Geometry check sheet. Reference: the model listing, model coordinates, mm. A direction names the side the tool comes from. Give positions to 0.01 mm unless a question says otherwise; leave off trailing zeros. Write each loop counter-clockwise with the first axis right and the second up, starting at its lowest first coordinate (ties: lowest second). Pieces come first, ordered by that corner, then holes. Notation, with made-up numbers: M 7.5,50 L 56.5,50 A23 ccw 56.5,78 Z; hole C 46,41.5 d10. An arc over 180 degrees is marked long. Write each question's results on one line, items separated by ' | '.
Autodesk Inventor part; units mm, degrees
ref_plane "YZ Plane" through (0, 0, 0) normal (1, 0, 0) x (0, 1, 0)
ref_plane "XZ Plane" through (0, 0, 0) normal (0, 1, 0) x (-1, 0, 0)
ref_plane "XY Plane" through (0, 0, 0) normal (0, 0, 1) x (1, 0, 0)
sketch "Sketch4" plane through (0, 0, 0) normal (0, 0, 1) x (1, 0, 0)
  line L0 (0, 500) -> (50, 500)
  line L1 (50, 500) -> (50, 0)
  line L2 (50, 0) -> (0, 0)
  line L3 (0, 0) -> (0, 500)
  dimension "d31" = 50
  dimension "d32" = 500
extrude "Extrusion1" add sketch "Sketch4" along normal blind 18.55
sketch "Sketch5" plane through (0, 0, 18.55) normal (0, 0, 1) x (1, 0, 0)
  line L0 (50, 500) -> (0, 500)
  line L1 (10, 500) -> (40, 500)
  line L2 (40, 500) -> (40, 537.1)
  line L3 (40, 537.1) -> (10, 537.1)
  line L4 (10, 537.1) -> (10, 500)
  line L5 (0, 500) -> (0, 0)
  line L6 (50, 0) -> (50, 500)
  dimension "d46" = 10
  dimension "d47" = 10
  dimension "d48" = 37.1
extrude "Extrusion2" add sketch "Sketch5" against normal blind 18.55
sketch "Sketch6" plane through (0, 0, 18.55) normal (0, 0, 1) x (1, 0, 0)
  line L0 (50, 500) -> (65, 491.3397)
  line L1 (65, 491.3397) -> (65, 486.3397)
  line L2 (65, 486.3397) -> (50, 486.3397)
  line L3 (50, 500) -> (40, 500)
  line L4 (40, 500) -> (50, 500)
  line L5 (50, 500) -> (50, 486.3397)
  line L6 (50, 0) -> (50, 500)
  line L7 (50, 475) -> (65, 466.3397)
  line L8 (65, 466.3397) -> (65, 461.3397)
  line L9 (65, 461.3397) -> (50, 461.3397)
  line L10 (50, 475) -> (50, 461.3397)
  line L11 (50, 450) -> (65, 441.3397)
  line L12 (65, 441.3397) -> (65, 436.3397)
  line L13 (65, 436.3397) -> (50, 436.3397)
  line L14 (50, 450) -> (50, 436.3397)
  line L15 (50, 425) -> (65, 416.3397)
  line L16 (65, 416.3397) -> (65, 411.3397)
  line L17 (65, 411.3397) -> (50, 411.3397)
  line L18 (50, 425) -> (50, 411.3397)
  line L19 (50, 400) -> (65, 391.3397)
  line L20 (65, 391.3397) -> (65, 386.3397)
  line L21 (65, 386.3397) -> (50, 386.3397)
  line L22 (50, 400) -> (50, 386.3397)
  line L23 (50, 375) -> (65, 366.3397)
  line L24 (65, 366.3397) -> (65, 361.3397)
  line L25 (65, 361.3397) -> (50, 361.3397)
  line L26 (50, 375) -> (50, 361.3397)
  line L27 (50, 350) -> (65, 341.3397)
  line L28 (65, 341.3397) -> (65, 336.3397)
  line L29 (65, 336.3397) -> (50, 336.3397)
  line L30 (50, 350) -> (50, 336.3397)
  line L31 (50, 325) -> (65, 316.3397)
  line L32 (65, 316.3397) -> (65, 311.3397)
  line L33 (65, 311.3397) -> (50, 311.3397)
  line L34 (50, 325) -> (50, 311.3397)
  line L35 (50, 300) -> (65, 291.3397)
  line L36 (65, 291.3397) -> (65, 286.3397)
  line L37 (65, 286.3397) -> (50, 286.3397)
  line L38 (50, 300) -> (50, 286.3397)
  line L39 (50, 275) -> (65, 266.3397)
  line L40 (65, 266.3397) -> (65, 261.3397)
  line L41 (65, 261.3397) -> (50, 261.3397)
  line L42 (50, 275) -> (50, 261.3397)
  line L43 (50, 250) -> (65, 241.3397)
  line L44 (65, 241.3397) -> (65, 236.3397)
  line L45 (65, 236.3397) -> (50, 236.3397)
  line L46 (50, 250) -> (50, 236.3397)
  line L47 (50, 225) -> (65, 216.3397)
  line L48 (65, 216.3397) -> (65, 211.3397)
  line L49 (65, 211.3397) -> (50, 211.3397)
  line L50 (50, 225) -> (50, 211.3397)
  line L51 (50, 200) -> (65, 191.3397)
  line L52 (65, 191.3397) -> (65, 186.3397)
  line L53 (65, 186.3397) -> (50, 186.3397)
  line L54 (50, 200) -> (50, 186.3397)
  line L55 (50, 175) -> (65, 166.3397)
  line L56 (65, 166.3397) -> (65, 161.3397)
  line L57 (65, 161.3397) -> (50, 161.3397)
  line L58 (50, 175) -> (50, 161.3397)
  line L59 (50, 150) -> (65, 141.3397)
  line L60 (65, 141.3397) -> (65, 136.3397)
  line L61 (65, 136.3397) -> (50, 136.3397)
  line L62 (50, 150) -> (50, 136.3397)
  line L63 (50, 125) -> (65, 116.3397)
  line L64 (65, 116.3397) -> (65, 111.3397)
  line L65 (65, 111.3397) -> (50, 111.3397)
  line L66 (50, 125) -> (50, 111.3397)
  line L67 (50, 100) -> (65, 91.3397)
  line L68 (65, 91.3397) -> (65, 86.3397)
  line L69 (65, 86.3397) -> (50, 86.3397)
  line L70 (50, 100) -> (50, 86.3397)
  line L71 (50, 75) -> (65, 66.3397)
  line L72 (65, 66.3397) -> (65, 61.3397)
  line L73 (65, 61.3397) -> (50, 61.3397)
  line L74 (50, 75) -> (50, 61.3397)
  line L75 (50, 50) -> (65, 41.3397)
  line L76 (65, 41.3397) -> (65, 36.3397)
  line L77 (65, 36.3397) -> (50, 36.3397)
  line L78 (50, 50) -> (50, 36.3397)
  line L79 (50, 25) -> (65, 16.3397)
  line L80 (65, 16.3397) -> (65, 11.3397)
  line L81 (65, 11.3397) -> (50, 11.3397)
  line L82 (50, 25) -> (50, 11.3397)
  point P0 (0, 0)
  point P1 (40, 475)
  point P2 (40, 450)
  point P3 (40, 425)
  point P4 (40, 400)
  point P5 (40, 375)
  point P6 (40, 350)
  point P7 (40, 325)
  point P8 (40, 300)
  point P9 (40, 275)
  point P10 (40, 250)
  point P11 (40, 225)
  point P12 (40, 200)
  point P13 (40, 175)
  point P14 (40, 150)
  point P15 (40, 125)
  point P16 (40, 100)
  point P17 (40, 75)
  point P18 (40, 50)
  point P19 (40, 25)
  dimension "d49" = 15
  dimension "d50" = 30
  dimension "d51" = 5
  dimension "d54" = 25
extrude "Extrusion3" add sketch "Sketch6" against normal blind 18.55 contours L75 L76 L77 L6 | L71 L72 L73 L6 | L67 L68 L69 L6 | L63 L64 L65 L6 | L59 L60 L61 L6 | L55 L56 L57 L6 | L51 L52 L53 L6 | L47 L48 L49 L6 | L43 L44 L45 L6 | L39 L40 L41 L6 | L35 L36 L37 L6 | L31 L32 L33 L6 | L27 L28 L29 L6 | L23 L24 L25 L6 | L19 L20 L21 L6 | L15 L16 L17 L6 | L11 L12 L13 L6 | L7 L8 L9 L6 | L0 L1 L2 L5
properties part number "graduated_foot"
Q1. Material ranges on probe 1 along Y at (x, z) = (49.5, 3.75); probe 2 along X at (y, z) = (285, 17); probe 3 along X at (y, z) = (503.5, 11.5), recorded low to high. Write a range as [from, to].
Answer key:
probe 1: y = [0, 500] | probe 2: x = [0, 50] | probe 3: x = [10, 40]
Q2. Section check A-A (y = 481.5). Enter the section's corners in (x, z), then the cut area to 4 significant figures.
Answer key:
outline: M 0,0 L 50,0 L 50,18.55 L 0,18.55 Z | area: 927.5 mm2
Q3. Depth check by flat-ended pin: P1, Ø5, axis at x = 6, z = 11, coming from the +Y side; P2, Ø10, axis at x = 44, z = 14, coming from the +Y side; P3, Ø3.5, axis at y = 279.5, z = 6.5, coming from the +X side; P4, Ø1.5, axis at x = 55, y = 310.5, coming from the +Z side. Enter the tip coordinate at first touch or a pass-through.
Answer key:
P1: stops at y = 500 | P2: stops at y = 537.1 | P3: stops at x = 50 | P4: passes through
Q4. Access from +Z, -Z, +X, -X, +Y, -Y to the whole of each face (thin tool, end or side, straight path). Record for faces 1 (the face through (5, 500, 9)), 2 (the face through (50, 18, 9)), 3 (the face through (57.395, 445.73, 9.405)).
Answer key:
face 1: +Z, -Z, -X, +Y | face 2: +Z, -Z, +X, -Y | face 3: +Z, -Z, +X
